The model under review builds one solid part; all positions refer to its coordinate system, in mm. Round coordinates to 2 decimals unless told otherwise and drop trailing zeros. Order: outer loops, then holes, each group sorted by start corner. A loop starts at its lowest first (then second) coordinate and runs counter-clockwise, first axis right, second up.
1) Consider section D-D (y = 51). Give the boundary of the cut face in (x, z), then the cut area to 3 significant figures.
2) To check wall thickness, follow L1, parallel to Y at x = 0, z = -1.5; L2, parallel to X at y = 11.5, z = -2.25; L3, parallel to Y at x = 40, z = -11.5. State the ranges of each line that lie inside material, in increasing order.
3) Consider section B-B (y = 0). Give the boundary of the cut face in (x, z).
4) Clearance check with flat-ended pins moving along their axes: P1, Ø3, axis at x = 0.5, z = -3, coming from the +Y side; P2, Ø5, axis at y = -51, z = 0, coming from the -X side; P3, Ø8, axis at y = -44.5, z = 10.5, coming from the +X side. State where each tip first meets the part, or that it passes through.
from build123d import *

# Parameters (mm, degrees)
SKETCH1_R           = 100
SKETCH1_R_2         = 25
BOSS_EXTRUDE1_DEPTH = 15
CUT_EXTRUDE1_DEPTH  = 12.5


with BuildPart() as part:
    # Sketch1 → Boss-Extrude1 (new, symmetric)
    with BuildSketch(Plane.XY):
        Circle(SKETCH1_R)
        Circle(SKETCH1_R_2, mode=Mode.SUBTRACT)
    extrude(amount=BOSS_EXTRUDE1_DEPTH, both=True)

    # Sketch2 → Cut-Extrude1 (cut, symmetric)
    with BuildSketch(Plane.XY):
        Polygon((100, 5), (110, -5), (100, -5), (60, -5), (60, 5), align=None)
        Polygon((45.961940777, -38.890872965), (74.246212025, -67.175144213), (74.246212025, -81.317279836), (67.175144213, -74.246212025), (38.890872965, -45.961940777), align=None)
        Polygon((5, -60), (5, -100), (-5, -110), (-5, -100), (-5, -60), align=None)
        Polygon((-38.890872965, -45.961940777), (-67.175144213, -74.246212025), (-81.317279836, -74.246212025), (-74.246212025, -67.175144213), (-45.961940777, -38.890872965), align=None)
        Polygon((-60, -5), (-100, -5), (-110, 5), (-100, 5), (-60, 5), align=None)
        Polygon((-45.961940777, 38.890872965), (-74.246212025, 67.175144213), (-74.246212025, 81.317279836), (-67.175144213, 74.246212025), (-38.890872965, 45.961940777), align=None)
        Polygon((-5, 60), (-5, 100), (5, 110), (5, 100), (5, 60), align=None)
        Polygon((38.890872965, 45.961940777), (67.175144213, 74.246212025), (81.317279836, 74.246212025), (74.246212025, 67.175144213), (45.961940777, 38.890872965), align=None)
    extrude(amount=CUT_EXTRUDE1_DEPTH, both=True, mode=Mode.SUBTRACT)


solid = part.part
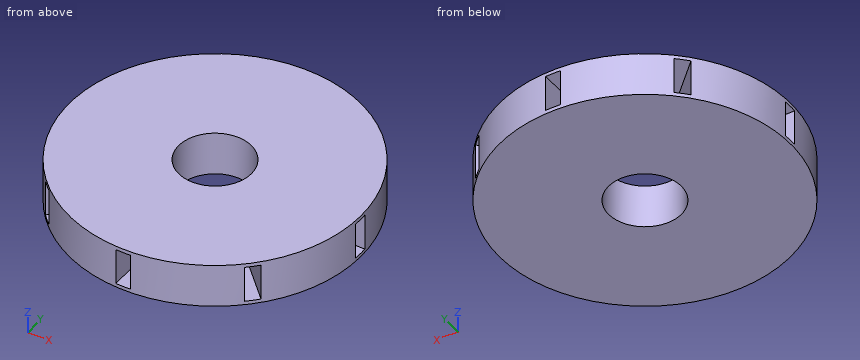
Answer below:
1. outline: (-86.02, -15) - (86.02, -15) - (86.02, 15) - (-86.02, 15) - close; hole (-58.07, -12.5) - (-43.93, -12.5) - (-43.93, 12.5) - (-58.07, 12.5) - close; hole (43.93, -12.5) - (58.07, -12.5) - (58.07, 12.5) - (43.93, 12.5) - close
1. area: 4,450 mm2
2. L1: y = -60 to -25, 25 to 60
2. L2: x = -99.34 to -22.2, 22.2 to 99.34
2. L3: y = -91.65 to -47.07, -44.85 to 44.85, 47.07 to 91.65
3. outline: (-100, -15) - (-25, -15) - (-25, 15) - (-100, 15) - (-100, 12.5) - (-60, 12.5) - (-60, -12.5) - (-100, -12.5) - close; (25, -15) - (100, -15) - (100, -12.5) - (60, -12.5) - (60, 12.5) - (100, 12.5) - (100, 15) - (25, 15) - close
4. P1: stops at y = 60
4. P2: stops at x = -87.45
4. P3: stops at x = 91.43
